The model under review builds one solid part; all positions refer to its coordinate system, in mm. A direction names the side the tool comes from. Give positions to 0.01 mm unless a question says otherwise; leave off trailing zeros. Loops run counter-clockwise (first coordinate to the right, second up) from the corner with the lowest first, then second, coordinate; pieces in that order, holes last. Notation, with made-up numbers: M 10.5,17 L 37.5,17 A31 ccw 37.5,43 Z; hole C 38.25,-4.75 d9. An arc over 180 degrees is marked long. Write item = value, one per line. Start each with the question number.
1. For faces 1 (the face through (-0.531, -1.857, 0.847)), 2 (the face through (-1, 0, -1)), list the 3-axis set-ups (+Z, -Z, +X, -X, +Y, -Y) from which the entire face can be reached by the end or side of a thin tool; tool diameter is ignored.
2. For pin 1 (1.5 mm diameter, centred on y = -3.5, z = 0.5, fed in from +X); pin 2 (2 mm diameter, centred on x = 0, y = -11, fed in from -Z); pin 3 (1 mm diameter, centred on y = -11, z = 1.5, fed in from -X); pin 4 (3 mm diameter, centred on x = 0.5, z = -2, fed in from -Y), all flat-tipped, find the tip position at first contact; note any pin that passes through.
3. Draft analysis for pull direction X (two halves, no side actions). For faces 3 (the face through (0, -25, 0)), 4 (the face through (0.556, -0.74, 1.007)), 5 (the face through (-0.07, -12.94, 1.5)), state which applies: pulls with the +X half, pulls with the -X half, needs draft (parallel to the pull), parting line crosses it, or undercut.
4. Wall thickness on line 1 along X through (y, z) = (-8.25, -0.05); line 2 along Y through (x, z) = (2.3, -1.05); line 3 along Y through (x, z) = (-2.05, 1.05): over which ranges is each line inside the solid? List them lowest first. Write a range as from..to.
5. We need section A-A on y = -17.5. Give the boundary of the cut face in (x, z).
Autodesk Inventor part; units mm, degrees
ref_plane "YZ Plane" through (0, 0, 0) normal (1, 0, 0) x (0, 1, 0)
ref_plane "XZ Plane" through (0, 0, 0) normal (0, 1, 0) x (-1, 0, 0)
ref_plane "XY Plane" through (0, 0, 0) normal (0, 0, 1) x (1, 0, 0)
sketch "Szkic2" plane through (0, 0, 0) normal (1, 0, 0) x (0, 1, 0)
  line L0 (0, -2.9) -> (0, 2.9)
  line L1 (-1.5, -1.5) -> (-1.5, 1.5)
  line L2 (-1.5, -1.5) -> (0, -2.9)
  line L3 (-1.5, 1.5) -> (0, 2.9)
  line L4 (0, 0) -> (-25, 0)
  line L5 (-25, 0) -> (-25, -1.5)
  line L6 (-25, -1.5) -> (-1.5, -1.5)
  dimension "d0" = 5.8
  dimension "d2" = 3
  dimension "d3" = 1.5
  dimension "d4" = 25
  dimension "d5" = 1.5
revolve "Obrót1" add sketch "Szkic2" angle 360 about axis through (0, 0, 0) along (0, -1, 0) contours L2 L1 L4 L0 | L6 L5 L4 L1
sketch "Szkic3" plane through (0, 0, 0) normal (0, 1, 0) x (1, 0, 0)
  line L0 (-1.1673, -0.633) -> (-1.1318, 0.6945)
  line L1 (-1.1318, 0.6945) -> (0.0355, 1.3274)
  line L2 (0.0355, 1.3274) -> (1.1673, 0.633)
  line L3 (1.1673, 0.633) -> (1.1318, -0.6945)
  line L4 (1.1318, -0.6945) -> (-0.0355, -1.3274)
  line L5 (-0.0355, -1.3274) -> (-1.1673, -0.633)
  point P0 (0, 0)
  point P1 (0, 0)
  dimension "d7" = 2.3
extrude "Wyciągnięcie proste1" cut sketch "Szkic3" against normal blind 2
fillet "Zaokrąglenie1" radius 0.5 6 edges at (-1.1496, -2, -0.0308) (-0.6014, -2, 0.9802) (-0.5482, -2, -1.011) (0.6014, -2, -0.9802) (0.5482, -2, 1.011) (1.1496, -2, 0.0308)
fillet "Zaokrąglenie2" radius 0.5 1 edges at (0, -1.5, 1.5)
fillet "Zaokrąglenie3" radius 0.1 1 edges at (0, 0, 2.9)
thread "Gwint1"
chamfer "Faza1" distance 0.5 angle 45 1 edges at (0, -25, 1.5)
properties part number "Screw M3 25mm flat head"
Final values:
q1.face_1 = +Y
q1.face_2 = +Z, -Z, +X, -X, +Y
q2.pin_1 = 1.5
q2.pin_2 = -1.5
q2.pin_3 = -1.12
q2.pin_4 = -25
q3.face_3 = needs draft
q3.face_4 = undercut
q3.face_5 = parting line crosses it
q4.line_1 = -1.5..1.5
q4.line_2 = -0.4..0
q4.line_3 = -0.64..0
q5.outline = C 0,0 d3
